Source: CAD feature listing. Evaluate the final solid. Frame: model axes, mm. A direction names the side the tool comes from. Round coordinates to 2 decimals unless told otherwise and drop trailing zeros. Order: outer loops, then holes, each group sorted by start corner. A loop starts at its lowest first (then second) coordinate and runs counter-clockwise, first axis right, second up. Notation, with made-up numbers: M 81.25,-9.75 L 130.25,-9.75 A25 cw 130.25,19.25 Z; hole C -22,50 d2. An arc over 180 degrees is marked long. Use one line per item in the form item = value. Start each with the question number.
Q1. Section A-A (z = -12). Return the cut outline in (x, y), plus the area to 3 significant figures.
Q2. Section C-C (x = -14.5). Return the cut outline in (y, z).
Q3. Reachability of faces 1 (the flat face through (-18, 1, -15)), 2 (the flat face through (14, 3, -22.5)), 3 (the flat face through (-14.2, 3, -22.5)) from +Z, -Z, +X, -X, +Y, -Y: full face, straight path, thin tool, end or side. Return the list, or none.
Q4. Material intervals for probe 1 along Y at (x, z) = (-16, -21); probe 2 along X at (y, z) = (11.25, -21.75); probe 3 along Z at (x, y) = (-9, 2.5), sorted ascending.
Q5. Contact query for flat-ended pins moving along their axis: pin 1 (0.8 mm diameter, centred on x = -16, z = -22.5, fed in from +Y); pin 2 (5 mm diameter, centred on x = -17.5, z = -14, fed in from +Y); pin 3 (5 mm diameter, centred on x = 13, y = 5, fed in from -Z); pin 4 (3.5 mm diameter, centred on y = 8.5, z = -22, fed in from -X). Output: stop coordinate, or through.
Q6. Section D-D (z = -8). Return the cut outline in (x, y).
Q7. Section B-B (y = 1.5). Return the cut outline in (x, z), plus the area to 3 significant figures.
Autodesk Fusion 360 part; units mm, degrees
sketch "Sketch1" plane through (0, 0, 0) normal (0, 1, 0) x (1, 0, 0) in component "Component"
  circle A0 centre (0, 0) radius 20.75
  line L0 (-22.5, 23) -> (22.5, 23)
  line L1 (0, 0) -> (0, 23) construction
  line L2 (-22.5, 23) -> (-22.5, 0)
  line L3 (22.5, 23) -> (22.5, 0)
  line L4 (-22.5, 0) -> (22.5, 0)
  line L5 (6.5, 19.7056) -> (6.5, 23)
  line L6 (-6.5, 19.7056) -> (-6.5, 23)
  line L7 (-22.5, 22) -> (22.5, 22)
  dimension "d1" = 41.5
  dimension "d2" = 45
  dimension "d3" = 23
  dimension "d4" = 13
  dimension "d9" = 1
extrude "Extrude1" add sketch "Sketch1" along normal blind 1 contours A0 L3 L4 L5 L7 | A0 L2 L4 L6 L7 | L0 L3 L5 L7 | L0 L2 L6 L7 makes body 1 at (13.5543, 0, -21.0541) makes body 2 at (-13.5543, 0, -21.0541) in component "Component"
extrude "Extrude2" add sketch "Sketch1" along normal blind 18 contours A0 L5 L6 L7 | L0 L5 L6 L7 bodies 1 2 in component "Component"
extrude "Extrude3" add sketch "Sketch1" along normal blind 3 contours L0 L3 L5 L7 | L0 L2 L6 L7 bodies 1 in component "Component"
fillet "Fillet1" radius 2 3 edges at (0, 18, -20.75) (6.5, 18, -21.3528) (-6.5, 18, -21.3528) on bodies 1 in component "Component"
fillet "Fillet2" radius 0.75 4 edges at (22.5, 0.5, 0) (-22.5, 0.5, 0) (22.5, 3, -22.5) (-22.5, 3, -22.5) on bodies 1 in component "Component"
fillet "Fillet3" radius 1 2 edges at (14.5, 1, -22) (-14.5, 1, -22) on bodies 1 in component "Component"
component "Component" placed x (1, 0, 0) y (0, 1, 0) z (0, 0, 1) at (0, 0, 0)
Results list:
q1.outline = M -22.5,0 L -16.93,0 L -16.93,1 L -22.5,1 Z; M 16.93,0 L 22.5,0 L 22.5,1 L 16.93,1 Z
q1.area = 11.1 mm2
q2.outline = M 0,-23 L 3,-23 L 3,-22 L 2,-22 A1 cw 1,-21 L 1,-14.84 L 0,-14.84 Z
q3.face_1 = +Z, -X, +Y
q3.face_2 = +Z, -Z, +X, +Y
q3.face_3 = +Z, -Z, -X, +Y
q4.probe_1 = 0 to 1
q4.probe_2 = -6.5 to 6.5
q4.probe_3 = -23 to -22
q5.pin_1 = 3
q5.pin_2 = 1
q5.pin_3 = -23
q5.pin_4 = -6.5
q6.outline = M -22.5,0 L -19.15,0 L -19.15,1 L -22.5,1 Z; M 19.15,0 L 22.5,0 L 22.5,1 L 19.15,1 Z
q7.outline = M -22.5,-23 L 22.5,-23 L 22.5,-21.87 L 6.5,-21.87 L 6.5,-19.71 A20.75 cw -6.5,-19.71 L -6.5,-21.87 L -22.5,-21.87 Z
q7.area = 70.0 mm2
